Design review of the part built by this model. Coordinates are the model's own, in mm. Face numbers are marked on the shaded views. A direction names the side the tool comes from. Round coordinates to 2 decimals unless told otherwise and drop trailing zeros. Loops run counter-clockwise (first coordinate to the right, second up) from the corner with the lowest first, then second, coordinate; pieces in that order, holes last. Notation, with made-up numbers: (17.5, 8) - (22.5, 8) arc R19 ccw to (22.5, 21) - close; hole circle Ø7 at (89, 52.25). An arc over 180 degrees is marked (long way). Return JSON: item names as keys, results as strings. Group by question number.
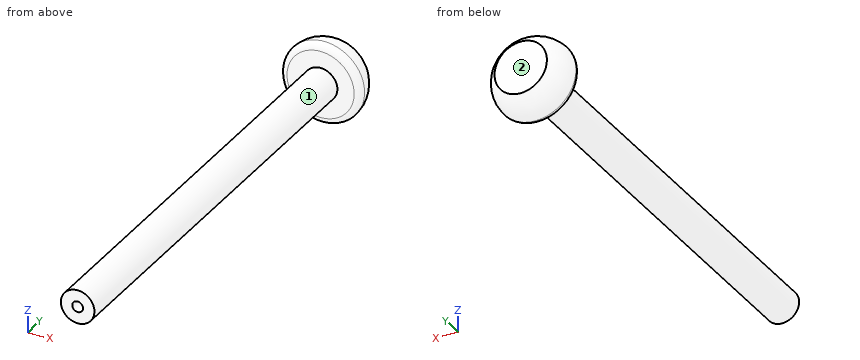
from build123d import *


with BuildPart() as part:
    # Esquisse1 → Révolution1 (revolve)
    with BuildSketch(Plane.XY, mode=Mode.PRIVATE) as r_volution1_sk:
        Polygon((8, 83.602856599), (8, 33.602856599), (25, 33.602856599), (25, 683.602856599), (0, 683.602856599), (0, 83.602856599), align=None)
        with BuildLine():
            Line((0, 693.602856599), (60, 693.602856599))
            ThreePointArc((60, 693.602856599), (54.2599688, 716.114995661), (38.965555337, 733.602856599))
            Line((38.965555337, 733.602856599), (0, 733.602856599))
            Line((0, 733.602856599), (0, 693.602856599))
        make_face()
        with BuildLine():
            Line((25, 683.602856599), (50, 683.602856599))
            ThreePointArc((50, 683.602856599), (57.071067812, 686.531788787), (60, 693.602856599))
            Line((60, 693.602856599), (0, 693.602856599))
            Line((0, 693.602856599), (0, 683.602856599))
            Line((0, 683.602856599), (25, 683.602856599))
        make_face()
    revolve(r_volution1_sk.sketch.rotate(Axis((0, -51.478862279, 0), (0, 1, 0)), 90), axis=Axis((0, -51.478862279, 0), (0, 1, 0)))


solid = part.part
Q1. Insertion check: pin 1 Ø4 at (x, z) = (-31, -8.5) entering from -Y; pin 2 Ø6 at (y, z) = (563, 25) entering from +X; pin 3 Ø3 at (y, z) = (335.5, 14) entering from -X. Each pin has a flat end and moves straight along its axis. Give the tip position at first contact, or say it passes through.
Q2. For line 1 (X direction, y = 51.5, z = 0); line 2 (Y direction, x = 11, z = 32); line 3 (X direction, y = 71, z = 19.5), list the stretches that pass through material, from the lowest coordinate up.
Q3. Tool access review of the marked faces 1 and 2: name each direction out of +Z, -Z, +X, -X, +Y, -Y from which nothing blocks a thin tool from reaching the whole face with its end or side.
Q4. Add section A-A, the plane y = 103. State the section outline as (x, z) points.
Evaluation:
{
 "1": {"pin 1": "y = 683.6", "pin 2": "x = 11.87", "pin 3": "x = -21.65"},
 "2": {"line 1": "-25 to -8, 8 to 25", "line 2": "683.6 to 733.6", "line 3": "-15.64 to 15.64"},
 "3": {"face 1": "-Y", "face 2": "+Z, -Z, +X, -X, +Y"},
 "4": {"outline": "circle Ø50 at (0, 0)"}
}
